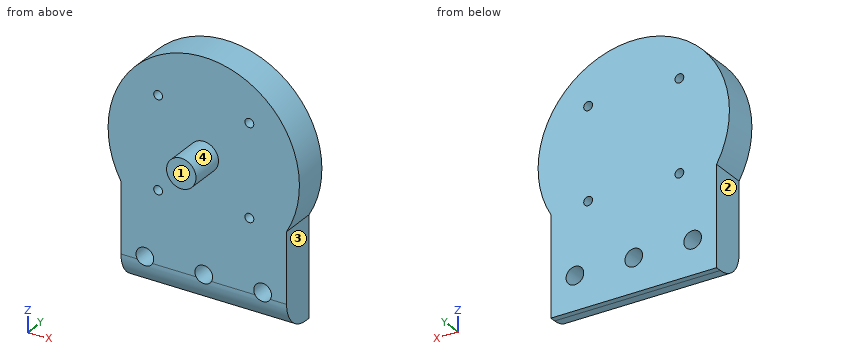
```python
from build123d import *

# Parameters (mm, degrees)
SKETCH_1_R          = 32.5
SKETCH_1_R_2        = 1.5
EXTRUDE_2_DEPTH     = 12
SKETCH_2_R          = 5
EXTRUDE_3_DEPTH     = 12
EXTRUDE_START       = -12
EXTRUDE_4_DEPTH     = 12
SKETCH_4_R          = 3
CUT_EXTRUDE_1_DEPTH = 12
FILLET_2_R          = 10


with BuildPart() as part:
    # 草图1 → 凸台-拉伸2 (new body)
    with BuildSketch(Plane(origin=(0, 0, 0), x_dir=(1, 0, 0), z_dir=(0, 1, 0))):
        with Locations(Location((0, 0, 0), (0, 0, 270))):
            Circle(SKETCH_1_R)
        with Locations(Location((-15.5, 15.5, 0), (0, 0, 270))):
            Circle(SKETCH_1_R_2, mode=Mode.SUBTRACT)
        with Locations(Location((15.5, 15.5, 0), (0, 0, 270))):
            Circle(SKETCH_1_R_2, mode=Mode.SUBTRACT)
        with Locations(Location((15.5, -15.5, 0), (0, 0, 270))):
            Circle(SKETCH_1_R_2, mode=Mode.SUBTRACT)
        with Locations(Location((-15.5, -15.5, 0), (0, 0, 270))):
            Circle(SKETCH_1_R_2, mode=Mode.SUBTRACT)
    extrude(amount=EXTRUDE_2_DEPTH)

    # 草图2 → 凸台-拉伸3 (add)
    with BuildSketch(Plane.XZ):
        with Locations(Location((0, 0, 0), (0, 0, 90))):
            Circle(SKETCH_2_R)
    extrude(amount=EXTRUDE_3_DEPTH)

    # 草图3 → 凸台-拉伸4 (add)
    with BuildSketch(Plane(origin=(0, 12, 0), x_dir=(1, 0, 0), z_dir=(0, 1, 0)).offset(EXTRUDE_START)):
        with BuildLine():
            Line((-28.145825623, 50), (-28.145825623, 16.25))
            ThreePointArc((-28.145825623, 16.25), (-16.25, 28.145825623), (0, 32.5))
            Line((0, 32.5), (0, 50))
            Line((0, 50), (-28.145825623, 50))
        make_face()
        with BuildLine():
            ThreePointArc((0, 32.5), (16.25, 28.145825623), (28.145825623, 16.25))
            Line((28.145825623, 16.25), (28.145825623, 50))
            Line((28.145825623, 50), (0, 50))
            Line((0, 50), (0, 32.5))
        make_face()
    extrude(amount=EXTRUDE_4_DEPTH)

    # 草图4 → 切除-拉伸1 (cut)
    with BuildSketch(Plane(origin=(0, 12, 0), x_dir=(1, 0, 0), z_dir=(0, 1, 0))):
        with Locations(Location((0, 38.5, 0), (0, 0, 270))):
            Circle(SKETCH_4_R)
        with Locations(Location((20, 38.5, 0), (0, 0, 270))):
            Circle(SKETCH_4_R)
        with Locations(Location((-20, 38.5, 0), (0, 0, 270))):
            Circle(SKETCH_4_R)
    extrude(amount=-CUT_EXTRUDE_1_DEPTH, mode=Mode.SUBTRACT)

    # 圆角2
    # the kernel refuses this fillet: 10 mm, written as the material it takes off along each edge
    with BuildSketch(Plane(origin=(53.145825623, 0, -50), x_dir=(0, 0, 1), z_dir=(-1, 0, 0))) as fillet_2_piece_1:
        with BuildLine():
            CenterArc((FILLET_2_R, FILLET_2_R), FILLET_2_R, 180, 90)
            Line((0, FILLET_2_R), (0, 0))
            Line((0, 0), (FILLET_2_R, 0))
        make_face()
    extrude(amount=106.291651246, mode=Mode.SUBTRACT)


solid = part.part
```
Can you work these out from the model? Positions are in its coordinate system, mm. Face numbers are marked on the shaded views. A direction names the side the tool comes from. Coordinates: 2 decimals unless noted, no trailing zeros. Loops run counter-clockwise (first coordinate to the right, second up) from the corner with the lowest first, then second, coordinate; pieces in that order, holes last.
1) Which directions (+Z, -Z, +X, -X, +Y, -Y) give clear straight access to the entire face, cutting with the end or side of a thin tool? Please do the marked faces 1, 2, 3 and 4.
2) Imagine slicing it at D-D on z = 15.5. List the corners of the cut face in (x, y) for me.
3) Imagine slicing it at A-A on z = -38.5. List the corners of the cut face in (x, y) for me.
4) For pin 1 (5 mm diameter, centred on x = -15.5, z = -15.5, fed in from -Y); pin 2 (3.5 mm diameter, centred on y = 8, z = -27, fed in from -X); pin 3 (12 mm diameter, centred on y = 9, z = 1.5, fed in from -X), each with a flat end and sliding along its axis, tell me the tip position at first contact or that it passes through.
5) Imagine slicing it at C-C on y = 2. List the corners of the cut face in (x, z) for me, plus the area to 3 significant figures.
6) Imagine slicing it at B-B on x = -20. List the corners of the cut face in (y, z) for me, plus the area to 3 significant figures.
7) I need wall thicknesses on probe 1 along X at (y, z) = (7.25, -38.5); probe 2 along X at (y, z) = (3, 15.5); probe 3 along Y at (x, z) = (-1, -11). Which ranges of each line are inside material? Lowest first, please.
Completed:
1. face 1: +Z, -Z, +X, -X, -Y
1. face 2: -Z, -X, +Y, -Y
1. face 3: -Z, +X, +Y, -Y
1. face 4: -Y
2. outline: (-28.57, 0) - (-17, 0) - (-17, 12) - (-28.57, 12) - close; (-14, 0) - (14, 0) - (14, 12) - (-14, 12) - close; (17, 0) - (28.57, 0) - (28.57, 12) - (17, 12) - close
3. outline: (-28.15, 0) - (-23, 0) - (-23, 12) - (-28.15, 12) - close; (-17, 0) - (-3, 0) - (-3, 12) - (-17, 12) - close; (3, 0) - (17, 0) - (17, 12) - (3, 12) - close; (23, 0) - (28.15, 0) - (28.15, 12) - (23, 12) - close
4. pin 1: stops at y = 0
4. pin 2: stops at x = -28.15
4. pin 3: stops at x = -32.5
5. outline: (-28.15, -46) - (28.15, -46) - (28.15, -16.25) arc R32.5 ccw (long way) to (-28.15, -16.25) - close; hole circle Ø6 at (-20, -38.5); hole circle Ø3 at (-15.5, -15.5); hole circle Ø3 at (-15.5, 15.5); hole circle Ø6 at (0, -38.5); hole circle Ø3 at (15.5, -15.5); hole circle Ø3 at (15.5, 15.5); hole circle Ø6 at (20, -38.5)
5. area: 4,230 mm2
6. outline: (0, -35.5) - (12, -35.5) - (12, 25.62) - (0, 25.62) - close; (0.11, -41.5) arc R10 ccw to (10, -50) - (12, -50) - (12, -41.5) - close
6. area: 814 mm2
7. probe 1: x = -28.15 to -23, -17 to -3, 3 to 17, 23 to 28.15
7. probe 2: x = -28.57 to -17, -14 to 14, 17 to 28.57
7. probe 3: y = 0 to 12
